```python
from build123d import *

# Parameters (mm, degrees)
BOSS_EXTRUDE1_REACH = 80.186
SKETCH3_R           = 2.5
BOSS_EXTRUDE2_REACH = 90.045
SKETCH4_R           = 2.5
SKETCH5_R           = 8.75
BOSS_EXTRUDE3_DEPTH = 2.7
BOSS_EXTRUDE4_START = -2.7
SKETCH6_R           = 8.75
BOSS_EXTRUDE4_DEPTH = 2.7
CUT_EXTRUDE1_REACH  = 90.045
SKETCH7_R           = 1.5


# Read off the part's stored shape, not the designer's step: Shell2
with BuildPart() as part:
    # Sketch1 → Revolve1 (revolve)
    with BuildSketch(Plane(origin=(0, 0, 0), x_dir=(1, 0, 0), z_dir=(0, 1, 0))):
        with BuildLine():
            Line((0, 29), (0, -29))
            ThreePointArc((0, -29), (-26, 0), (0, 29))
        make_face()
    revolve(axis=Axis((0, 0, -29), (0, 0, 1)))

    # Sketch3 → Boss-Extrude1 (add, up to next)
    with BuildSketch(Plane.XY.offset(40), mode=Mode.PRIVATE) as boss_extrude1_sk1:
        Circle(SKETCH3_R)
    boss_extrude1_tool1 = extrude(boss_extrude1_sk1.sketch, amount=-BOSS_EXTRUDE1_REACH, mode=Mode.PRIVATE) - part.part
    add(boss_extrude1_tool1.solids().sort_by_distance((0, 0, 40))[0])

    # Sketch4 → Boss-Extrude2 (add, up to next)
    with BuildSketch(Plane.XY.offset(-40), mode=Mode.PRIVATE) as boss_extrude2_sk1:
        Circle(SKETCH4_R)
    boss_extrude2_tool1 = extrude(boss_extrude2_sk1.sketch, amount=BOSS_EXTRUDE2_REACH, mode=Mode.PRIVATE) - part.part
    add(boss_extrude2_tool1.solids().sort_by_distance((0, 0, -40))[0])

    # Shell2 outline → Shell2 (revolve, cut)
    with BuildSketch(Plane.XZ):
        with BuildLine():
            Line((1, 27.356619224), (1, 40))
            Line((1, 40), (0, 40))
            Line((0, 40), (0, -38.5))
            Line((0, -38.5), (1, -38.5))
            Line((1, -38.5), (1, -27.356619224))
            ThreePointArc((1, -27.356619224), (24.5, 0), (1, 27.356619224))
        make_face()
    revolve(axis=Axis((0, 0, 0), (0, 0, 1)), mode=Mode.SUBTRACT)

    # Sketch5 → Boss-Extrude3 (add)
    with BuildSketch(Plane.XY.offset(40)):
        Circle(SKETCH5_R)
    extrude(amount=-BOSS_EXTRUDE3_DEPTH)

    # Sketch6 → Boss-Extrude4 (add)
    with BuildSketch(Plane(origin=(0, 0, -40), x_dir=(-1, 0, 0), z_dir=(0, 0, -1)).offset(BOSS_EXTRUDE4_START)):
        with Locations(Location((0, 0, 0), (0, 0, 180))):
            Circle(SKETCH6_R)
    extrude(amount=BOSS_EXTRUDE4_DEPTH)

    # Sketch7 → Cut-Extrude1 (cut, up to next)
    with BuildSketch(Plane.XY.offset(40), mode=Mode.PRIVATE) as cut_extrude1_sk1:
        Circle(SKETCH7_R)
    cut_extrude1_tool1 = extrude(cut_extrude1_sk1.sketch, amount=-CUT_EXTRUDE1_REACH, mode=Mode.PRIVATE) & part.part
    add(cut_extrude1_tool1.solids().sort_by_distance((0, 0, 40))[0], mode=Mode.SUBTRACT)


solid = part.part
```
The listing builds one solid part. Answer for the finished solid, in the listing's coordinates (mm). A direction names the side the tool comes from. Round coordinates to 2 decimals unless told otherwise and drop trailing zeros. Loops run counter-clockwise (first coordinate to the right, second up) from the corner with the lowest first, then second, coordinate; pieces in that order, holes last. Notation, with made-up numbers: (84.5, 23.25) -> (105.5, 23.25) arc R30 ccw to (105.5, 54.25) -> close; hole circle Ø3 at (-29, 82). An arc over 180 degrees is marked (long way). Use one line per item in the form item = value.
1. Flat-ended cylindrical pins translate along their axes: pin 1 Ø4 at (y, z) = (-15, -13) entering from +X; pin 2 Ø8 at (y, z) = (8, 15.5) entering from -X; pin 3 Ø1.5 at (x, z) = (-16.5, 7) entering from +Y; pin 4 Ø3.5 at (x, y) = (0, 0) entering from +Z. Find the tip coordinate at first contact, or state that the pin passes through.
Answer key:
pin_1 = 19.31
pin_2 = -22.62
pin_3 = 19.65
pin_4 = 40
2. A tool of negligible diameter and unlimited length cuts with its end or side. For faces 1 (the flat face through (0, -2, 40)), 2 (the flat face through (2, -2, 37.3)), 3 (the cylindrical face through (-6.944, -5.324, 38.669)), from which of +Z, -Z, +X, -X, +Y, -Y can it reach the whole face along a straight path? Write none if from no direction.
Answer key:
face_1 = +Z, +X, -X, +Y, -Y
face_2 = none
face_3 = +Z
3. The part is cut by section B-B on y = -7.5. Give the number of separate pieces and of enclosed holes in the cut face, and give its area (3 significant figures).
Answer key:
separate_pieces = 3
enclosed_holes = 1
area = 298 mm²
4. Find the intervals of material crossed by probe 1 along Y at (x, z) = (0, 35.25); probe 2 along Y at (x, z) = (0, -29), in increasing order. Write a range as [from, to].
Answer key:
probe_1 = [-2.5, -1.5], [1.5, 2.5]
probe_2 = [-2.5, -1], [1, 2.5]
5. The part is cut by section A-A on z = 33.5. Determine the outline of the cut face in (x, y).
Answer key:
outline = circle Ø5 at (0, 0); hole circle Ø3 at (0, 0)
6. For a pull along Z with two mould halves and no side action, classify faces 4 (the cylindrical face through (-0.54, -2.44, -33.02)), 5 (the cylindrical face through (-1.9, 8.54, -38.63)), 6 (the flat face through (0, 0, -37.3)) as released by +Z, released by -Z, zero draft, split by the parting line, or undercut.
Answer key:
face_4 = undercut
face_5 = zero draft
face_6 = released by +Z
